Geometry: see drawing. Coordinates: mm, zero at the bounding-box minimum. A direction names the side the tool comes from. Coordinates: 2 decimals unless noted, no trailing zeros. Write each loop counter-clockwise with the first axis right and the second up, starting at its lowest first coordinate (ties: lowest second). Pieces come first, ordered by that corner, then holes. Notation, with made-up numbers: (1.5, 84) - (6.5, 84) arc R24 ccw to (6.5, 96) - close; hole circle Ø3 at (31.5, 50). An arc over 180 degrees is marked (long way). Use a Markdown table: item, result. Add a question column.
Q1. Material intervals for probe 1 along Y at (x, z) = (5, 1.4); probe 2 along X at (y, z) = (101, 28); probe 3 along Y at (x, z) = (69.5, 19.5), sorted ascending. Write a range as from..to.
Q2. Section query B-B (z = 3.5). Return the cut outline in (x, y).
Q3. Pin query (flat end, axial travel): P1, Ø1.5, axis at y = 44.5, z = 5, coming from the -X side; P2, Ø5, axis at x = 35.5, z = 23, coming from the -Y side; P3, Ø8, axis at x = 5.5, y = 45.5, coming from the +Z side. Return the tip coordinate at first contact, or that it passes through.
Q4. Mould query, pull axis X, two halves, no side actions, for the marked faces 1, 2 and 3. Classes: released by +X, released by -X, zero draft, split by the parting line, or undercut.
Q5. Section query C-C (x = 5). Return the cut outline in (y, z), then the cut area to 3 significant figures.
Q6. Set-up query: the marked faces 4 and 5. Return all of +Z, -Z, +X, -X, +Y, -Y with unobstructed straight access to the full face (end or side cutting, diameter ignored); none if empty.
Q7. Section query A-A (y = 85). Return the cut outline in (x, z), then the cut area to 3 significant figures.
Q8. Section query D-D (x = 62). Return the cut outline in (y, z), then the cut area to 3 significant figures.
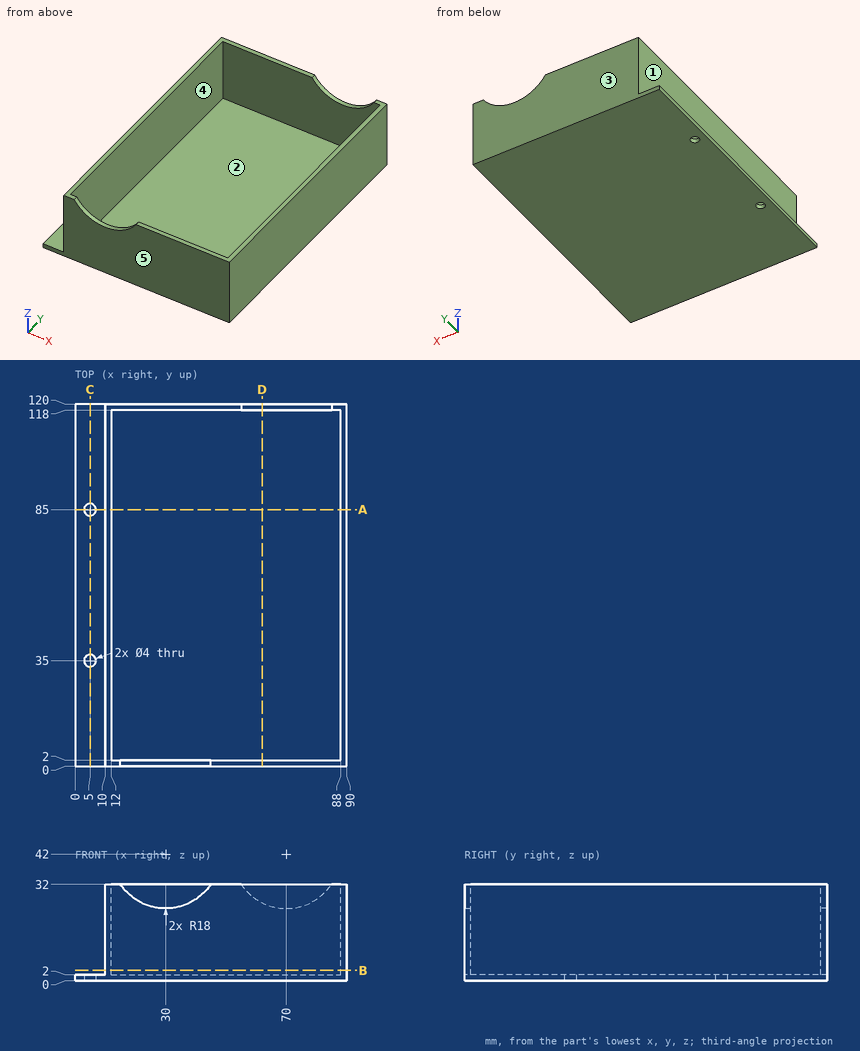
Values follow:
| question | item | result |
|---|---|---|
| 1 | probe 1 | 0..33, 37..83, 87..120 |
| 1 | probe 2 | 10..12, 88..90 |
| 1 | probe 3 | 0..2, 118..120 |
| 2 | outline | (10, 0) - (90, 0) - (90, 120) - (10, 120) - close; hole (12, 2) - (88, 2) - (88, 118) - (12, 118) - close |
| 3 | P1 | x = 10 |
| 3 | P2 | y = 0 |
| 3 | P3 | z = 2 |
| 4 | face 1 | released by -X |
| 4 | face 2 | undercut |
| 4 | face 3 | zero draft |
| 5 | outline | (0, 0) - (33, 0) - (33, 2) - (0, 2) - close; (37, 0) - (83, 0) - (83, 2) - (37, 2) - close; (87, 0) - (120, 0) - (120, 2) - (87, 2) - close |
| 5 | area | 224 mm2 |
| 6 | face 4 | +Z |
| 6 | face 5 | +Z, -Z, +X, -X, -Y |
| 7 | outline | (0, 0) - (3, 0) - (3, 2) - (0, 2) - close; (7, 0) - (90, 0) - (90, 32) - (88, 32) - (88, 2) - (12, 2) - (12, 32) - (10, 32) - (10, 2) - (7, 2) - close |
| 7 | area | 292 mm2 |
| 8 | outline | (0, 0) - (120, 0) - (120, 25.88) - (118, 25.88) - (118, 2) - (2, 2) - (2, 32) - (0, 32) - close |
| 8 | area | 348 mm2 |
